```python
from build123d import *

# Parameters (mm, degrees)
SKETCH1_W                      = 60
SKETCH1_H                      = 450
BASE_FLANGE1_DEPTH             = 1
EDGE_FLANGE1_STRIP_W           = 5.4732
EDGE_FLANGE1_STRIP_H           = 1
EDGE_FLANGE1_STRIP_CUT_DEPTH   = 450
EDGE_FLANGE1_STRIP_2_W         = 5.4732
EDGE_FLANGE1_STRIP_2_H         = 1
EDGE_FLANGE1_STRIP_CUT_2_DEPTH = 450
EDGE_FLANGE1_DEPTH             = 450
EDGE_FLANGE1_BEND_DEPTH        = 450


# Sheet-metal steps are written as plain solids
with BuildPart() as part:
    # Sketch1 → Base-Flange1 (new body)
    with BuildSketch(Plane.XY):
        Rectangle(SKETCH1_W, SKETCH1_H)
    extrude(amount=-BASE_FLANGE1_DEPTH)

    # Edge-Flange1 strip (across the edge) → Edge-Flange1 strip cut (cut)
    with BuildSketch(Plane(origin=(30, -225, 0), x_dir=(-1, 0, 0), z_dir=(0, 1, 0))):
        with Locations((-1, -0.5)):
            Rectangle(EDGE_FLANGE1_STRIP_W, EDGE_FLANGE1_STRIP_H)
    extrude(amount=EDGE_FLANGE1_STRIP_CUT_DEPTH, mode=Mode.SUBTRACT)

    # Edge-Flange1 strip 2 (across the edge) → Edge-Flange1 strip cut 2 (cut)
    with BuildSketch(Plane(origin=(-30, 225, 0), x_dir=(1, 0, 0), z_dir=(0, -1, 0))):
        with Locations((-1, -0.5)):
            Rectangle(EDGE_FLANGE1_STRIP_2_W, EDGE_FLANGE1_STRIP_2_H)
    extrude(amount=EDGE_FLANGE1_STRIP_CUT_2_DEPTH, mode=Mode.SUBTRACT)

    # Edge-Flange1 section (across the edge) → Edge-Flange1 (add)
    with BuildSketch(Plane(origin=(30, -225, 0), x_dir=(-1, 0, 0), z_dir=(0, 1, 0))):
        with BuildLine():
            Line((0, 0.7366), (0, 14))
            Line((0, 14), (1, 14))
            Line((1, 14), (1, 0.7366))
            ThreePointArc((1, 0.7366), (1.215745145, 0.215745145), (1.7366, 0))
            Line((1.7366, 0), (1.7366, -1))
            ThreePointArc((1.7366, -1), (0.508638364, -0.491361636), (0, 0.7366))
        make_face()
    extrude(amount=EDGE_FLANGE1_DEPTH)

    # Edge-Flange1 section 2 (across the edge) → Edge-Flange1 bend (add)
    with BuildSketch(Plane(origin=(-30, 225, 0), x_dir=(1, 0, 0), z_dir=(0, -1, 0))):
        with BuildLine():
            Line((0, 0.7366), (0, 14))
            Line((0, 14), (1, 14))
            Line((1, 14), (1, 0.7366))
            ThreePointArc((1, 0.7366), (1.215745145, 0.215745145), (1.7366, 0))
            Line((1.7366, 0), (1.7366, -1))
            ThreePointArc((1.7366, -1), (0.508638364, -0.491361636), (0, 0.7366))
        make_face()
    extrude(amount=EDGE_FLANGE1_BEND_DEPTH)


solid = part.part
```
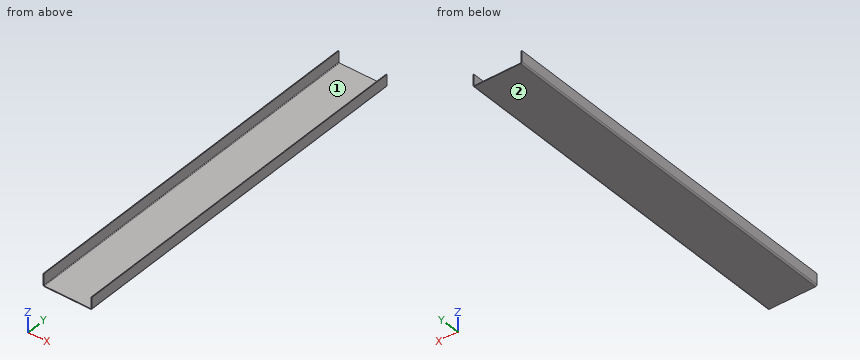
The listing builds one solid part. Answer for the finished solid, in the listing's coordinates (mm). Face numbers are marked on the shaded views. Coordinates: 2 decimals unless noted, no trailing zeros. Loops run counter-clockwise (first coordinate to the right, second up) from the corner with the lowest first, then second, coordinate; pieces in that order, holes last. Notation, with made-up numbers: M 75,4.25 L 97,4.25 A28 cw 97,38.25 Z; hole C 41.5,48 d10. An arc over 180 degrees is marked long. Answer as CSV lines item,"result". Start each with the question number.
(1) The part is cut by section B-B (y = -69). Give the vertices of the cut face in (x, z), and give its area (3 significant figures).
(2) The part is cut by section C-C (x = -9). Give the vertices of the cut face in (y, z), and give its area (3 significant figures).
(3) Given pin 1 (2 mm diameter, centred on x = -5.5, y = -33, fed in from +Z), flat-ended and moving along its own axis, determine where the tip first touches the part or whether it passes through.
(4) The mould has two halves that part along X. Classify the marked faces 1 and 2: pulls with the +X half, pulls with the -X half, needs draft (parallel to the pull), parting line crosses it, or undercut.
(5) The part is cut by section A-A (z = 10.5). Give the vertices of the cut face in (x, y).
(6) Find the intervals of material crossed by L1, parallel to X at y = -169, z = 8.25; L2, parallel to Z at x = -20, y = 101; L3, parallel to X at y = -55.5, z = -0.25, in increasing order. Write a range as [from, to].
Determined:
1,outline,"M -30,0.74 A1.74 ccw -28.26,-1 L 28.26,-1 A1.74 ccw 30,0.74 L 30,14 L 29,14 L 29,0.74 A0.74 cw 28.26,0 L -28.26,0 A0.74 cw -29,0.74 L -29,14 L -30,14 Z"
1,area,"86.9 mm2"
2,outline,"M -225,-1 L 225,-1 L 225,0 L -225,0 Z"
2,area,"450 mm2"
3,pin 1,"z = 0"
4,face 1,"undercut"
4,face 2,"needs draft"
5,outline,"M -30,-225 L -29,-225 L -29,225 L -30,225 Z; M 29,-225 L 30,-225 L 30,225 L 29,225 Z"
6,L1,"[-30, -29], [29, 30]"
6,L2,"[-1, 0]"
6,L3,"[-29.69, 29.69]"
